```python
from build123d import *

# Parameters (mm, degrees)
F0_W      = 64
F0_H      = 38
F0_W_2    = 50
F0_H_2    = 28.5
F1_DEPTH  = 30
F3_D      = 2
F3_DEPTH  = 15
F3_TIP    = 0.600860619
F4_W      = 64
F4_H      = 38
F5_DEPTH  = 3
F6_W      = 10
F6_H      = 28.5
F8_DEPTH  = 15.75
F10_DEPTH = 38
F11_R     = 2
F13_DEPTH = 3
F15_D     = 2


with BuildPart() as f1:
    # F0 (on Top) → F1 (new body)
    with BuildSketch(Plane.XY):
        with Locations((32, 19)):
            Rectangle(F0_W, F0_H)
        with Locations((32, 17.25)):
            Rectangle(F0_W_2, F0_H_2, mode=Mode.SUBTRACT)
    extrude(amount=F1_DEPTH)

    # F3
    with Locations(Plane(origin=(0, 0, 0), x_dir=(1, 0, 0), z_dir=(0, 0, -1))):
        with Locations((2.5, -2.5), (61.5, -2.5), (61.5, -35.5), (2.5, -35.5)):
            Hole(F3_D / 2, depth=F3_DEPTH)
            with Locations((0, 0, -(F3_DEPTH + F3_TIP / 2))):  # 118° drill point
                Cone(0, F3_D / 2, F3_TIP, mode=Mode.SUBTRACT)

    # F4 (on face) → F5 (join)
    with BuildSketch(Plane.XY.offset(30)):
        with Locations((32, 19)):
            Rectangle(F4_W, F4_H)
    extrude(amount=F5_DEPTH)

    # F6 (on face) → F8 (join, through all)
    with BuildSketch(Plane(origin=(0, 0, 30), x_dir=(1, 0, 0), z_dir=(0, 0, -1))):
        with Locations((12, -17.25)):
            Rectangle(F6_W, F6_H)
    extrude(amount=F8_DEPTH)

    # F9 (on face) → F10 (cut, through all)
    with BuildSketch(Plane.XZ):
        Polygon((0, 33), (0, 15), (5, 33), align=None)
        Polygon((64, 33), (59, 33), (64, 15), align=None)
    extrude(amount=-F10_DEPTH, mode=Mode.SUBTRACT)

    # F11
    f11_edges = [f1.edges().sort_by_distance(p)[0] for p in [
        (0, 0, 7.5),
        (2.5, 0, 24),
        (61.5, 0, 24),
        (64, 0, 7.5),
        (2.5, 38, 24),
        (0, 38, 7.5),
        (64, 38, 7.5),
        (61.5, 38, 24),
        (32, 0, 33),
        (5, 19, 33),
        (32, 38, 33),
        (59, 19, 33),
    ]]
    fillet(f11_edges, radius=F11_R)

    # F12 (on face) → F13 (cut, through all)
    with BuildSketch(Plane.XZ):
        with BuildLine():
            Line((28.9344657888, 16.05), (35.0655342112, 16.05))
            ThreePointArc((35.0655342112, 16.05), (32, 25), (28.9344657888, 16.05))
        make_face()
    extrude(amount=-F13_DEPTH, mode=Mode.SUBTRACT)

    # F15 (through all)
    with Locations(Plane.XY.offset(33)):
        with Locations((27, 19), (37, 19)):
            Hole(F15_D / 2)


solid = f1.part
```
For this review, take the finished solid that the model builds, in its own axes (mm). A direction names the side the tool comes from. Give positions to 0.01 mm unless a question says otherwise; leave off trailing zeros. Write each loop counter-clockwise with the first axis right and the second up, starting at its lowest first coordinate (ties: lowest second). Pieces come first, ordered by that corner, then holes. Notation, with made-up numbers: M 20,27 L 63,27 A18 cw 63,62 Z; hole C 57,30 d8. An arc over 180 degrees is marked long. Answer as a JSON object with one key per item and string values. Group by question number.
Item 1: For pin 1 Ø8 at (y, z) = (9.5, 27) entering from +X; pin 2 Ø1.6 at (x, y) = (27, 19) entering from -Z; pin 3 Ø1.2 at (x, y) = (61.5, 2.5) entering from -Z; pin 4 Ø6 at (x, z) = (32, 20) entering from -Y, all flat-tipped, find the tip position at first contact; note any pin that passes through.
Item 2: Consider section A-A on y = 19. Write out the cut boundary in (x, z).
Item 3: Draft analysis for pull direction Z (two halves, no side actions). For faces 3 (the cylindrical face through (32, 1, 25)), 4 (the flat face through (57, 17, 15)), 5 (the cylindrical face through (32.36, 0.57, 32.4)), state which applies: +Z half, -Z half, draft (parallel to the pull), parting line (faces both ways), or undercut.
Item 4: Consider section B-B on x = 32. Write out the cut boundary in (y, z).
Item 5: For probe 1 along X at (y, z) = (35.5, 9.75); probe 2 along Y at (x, z) = (61.5, 6.25); probe 3 along Y at (x, z) = (49, 4.5), list the stretches that pass through material, from the lowest coordinate up. Write a range as [from, to].
Item 6: Tool access review of faces 1 (the cylindrical face through (3.3, 3.1, 7.6)), 2 (the flat face through (32, 38, 15)): name each direction out of +Z, -Z, +X, -X, +Y, -Y from which nothing blocks a thin tool from reaching the whole face with its end or side.
Item 7: Consider section C-C on z = 11.5. Write out the cut boundary in (x, y).
Item 8: Consider section D-D on x = 12. Write out the cut boundary in (y, z), plus the area to 3 significant figures.
Check result:
{
 "1": {"pin 1": "stops at x = 61.78", "pin 2": "passes through", "pin 3": "stops at z = 15.24", "pin 4": "stops at y = 31.5"},
 "2": {"outline": "M 0,0 L 7,0 L 7,14.25 L 17,14.25 L 17,30 L 26,30 L 26,33 L 6.52,33 A2 ccw 4.59,31.54 L 0,15 Z; M 28,30 L 36,30 L 36,33 L 28,33 Z; M 38,30 L 57,30 L 57,0 L 64,0 L 64,15 L 59.41,31.54 A2 ccw 57.48,33 L 38,33 Z"},
 "3": {"face 3": "undercut", "face 4": "draft", "face 5": "+Z half"},
 "4": {"outline": "M 0,0 L 3,0 L 3,16.05 L 0,16.05 Z; M 0,25 L 3,25 L 3,30 L 31.5,30 L 31.5,0 L 38,0 L 38,31 A2 ccw 36,33 L 2,33 A2 ccw 0,31 Z"},
 "5": {"probe 1": "x = [0, 1.5], [3.5, 60.5], [62.5, 64]", "probe 2": "y = [0, 1.5], [3.5, 34.5], [36.5, 38]", "probe 3": "y = [0, 3], [31.5, 38]"},
 "6": {"face 1": "-Z", "face 2": "+Z, -Z, +X, -X, +Y"},
 "7": {"outline": "M 0,2 A2 ccw 2,0 L 62,0 A2 ccw 64,2 L 64,36 A2 ccw 62,38 L 2,38 A2 ccw 0,36 Z; hole C 2.5,2.5 d2; hole C 2.5,35.5 d2; hole M 7,3 L 57,3 L 57,31.5 L 7,31.5 Z; hole C 61.5,2.5 d2; hole C 61.5,35.5 d2"},
 "8": {"outline": "M 0,0 L 3,0 L 3,14.25 L 31.5,14.25 L 31.5,0 L 38,0 L 38,31 A2 ccw 36,33 L 2,33 A2 ccw 0,31 Z", "area": "846 mm^2"}
}
